Read the model definition and answer for the solid it produces. Units are mm, in the model's axes. A direction names the side the tool comes from. Coordinates: 2 decimals unless noted, no trailing zeros. Order: outer loops, then holes, each group sorted by start corner. A loop starts at its lowest first (then second) coordinate and runs counter-clockwise, first axis right, second up. Notation, with made-up numbers: M 35,-31 L 46,-31 A22 cw 46,-12 Z; hole C 45.5,68.5 d5. An arc over 180 degrees is marked long. Write each question's results on one line, items separated by ' | '.
```python
from build123d import *

# Parameters (mm, degrees)
BOSS_EXTRUDE1_DEPTH = 70
CUT_EXTRUDE1_DEPTH  = 65
SKETCH5_W           = 80
SKETCH5_H           = 35
BOSS_EXTRUDE2_DEPTH = 18
SKETCH6_W           = 70
SKETCH6_H           = 25
CUT_EXTRUDE2_DEPTH  = 18


with BuildPart() as part:
    # Sketch1 → Boss-Extrude1 (new body)
    with BuildSketch(Plane(origin=(0, 0, 0), x_dir=(1, 0, 0), z_dir=(0, 1, 0))):
        Polygon((-55.37403033, -102.482648945), (3.252686078, -116.449526131), (57.060212297, -100.408827863), (76.3, -57.735026919), (-76.3, -57.735026919), align=None)
    extrude(amount=BOSS_EXTRUDE1_DEPTH)

    # Sketch4 → Cut-Extrude1 (cut)
    with BuildSketch(Plane(origin=(0, 70, 0), x_dir=(1, 0, 0), z_dir=(0, 1, 0))):
        Polygon((-51.867290581, -98.178143042), (3.108154981, -111.275163368), (53.44146669, -96.270172009), (71.3, -57.735026919), (-71.3, -57.735026919), align=None)
    extrude(amount=-CUT_EXTRUDE1_DEPTH, mode=Mode.SUBTRACT)

    # Sketch5 → Boss-Extrude2 (add)
    with BuildSketch(Plane.XY.offset(117)):
        with Locations((3.252686078, 35)):
            Rectangle(SKETCH5_W, SKETCH5_H)
    extrude(amount=-BOSS_EXTRUDE2_DEPTH)

    # Sketch6 → Cut-Extrude2 (cut)
    with BuildSketch(Plane.XY.offset(117)):
        with Locations((3.252686078, 35)):
            Rectangle(SKETCH6_W, SKETCH6_H)
    extrude(amount=-CUT_EXTRUDE2_DEPTH, mode=Mode.SUBTRACT)


solid = part.part
```
(1) The part is cut by section A-A, the plane y = 28. Write down the section's boundary in (x, z).
Conclusion:
outline: M -76.3,57.74 L -71.3,57.74 L -51.87,98.18 L -36.75,101.78 L -36.75,99 L -31.75,99 L -31.75,117 L -36.75,117 L -36.75,106.92 L -55.37,102.48 Z; M 38.25,99 L 43.25,99 L 43.25,99.31 L 53.44,96.27 L 71.3,57.74 L 76.3,57.74 L 57.06,100.41 L 43.25,104.53 L 43.25,117 L 38.25,117 Z
(2) The mould has two halves that part along X. Classify faces 5 (the flat face through (47.7, 34.5, 103.2)), 6 (the flat face through (-39.499, 34.51, 106.265)), 7 (the flat face through (0, 22, 99)), 8 (the flat face through (62.246, 37.955, 77.272)): pulls with the +X half, pulls with the -X half, needs draft (parallel to the pull), parting line crosses it, or undercut.
Conclusion:
face 5: pulls with the +X half | face 6: pulls with the -X half | face 7: undercut | face 8: undercut
(3) For faces 1 (the flat face through (3, 52.5, 104)), 2 (the flat face through (3, 17.5, 104)), 3 (the flat face through (43.253, 35, 111)), 4 (the flat face through (3, 47.5, 108)), determine the directions among +Z, -Z, +X, -X, +Y, -Y from which every point of the face is accessible in a straight line to the end or side of a thin tool.
Conclusion:
face 1: -Z, +Y | face 2: -Z | face 3: +Z, +X, +Y, -Y | face 4: +Z, -Z
(4) The part is cut by section B-B, the plane x = 17.5. Write down the section's boundary in (y, z), then the cut area to 3 significant figures.
Conclusion:
outline: M 0,57.74 L 5,57.74 L 5,106.98 L 17.5,106.98 L 17.5,99 L 22.5,99 L 22.5,117 L 17.5,117 L 17.5,112.2 L 0,112.2 Z; M 47.5,99 L 52.5,99 L 52.5,106.98 L 70,106.98 L 70,112.2 L 52.5,112.2 L 52.5,117 L 47.5,117 Z | area: 609 mm²
(5) The part is cut by section C-C, the plane z = 109. Write down the section's boundary in (x, y).
Conclusion:
outline: M -36.75,17.5 L -28.02,17.5 L -28.02,0 L 28.24,0 L 28.24,17.5 L 43.25,17.5 L 43.25,52.5 L 28.24,52.5 L 28.24,70 L 10.74,70 L 10.74,52.5 L -6.44,52.5 L -6.44,70 L -28.02,70 L -28.02,52.5 L -36.75,52.5 Z; hole M -31.75,22.5 L 38.25,22.5 L 38.25,47.5 L -31.75,47.5 Z; hole M -6.44,5 L 10.74,5 L 10.74,17.5 L -6.44,17.5 Z
(6) The part is cut by section D-D, the plane y = 12. Write down the section's boundary in (x, z).
Conclusion:
outline: M -76.3,57.74 L -71.3,57.74 L -51.87,98.18 L 3.11,111.28 L 53.44,96.27 L 71.3,57.74 L 76.3,57.74 L 57.06,100.41 L 3.25,116.45 L -55.37,102.48 Z
(7) Straight lines are drawn through the part: line 1 (Y direction, x = 0, z = 105); line 2 (Y direction, x = 12, z = 112); line 3 (X direction, y = 40.5, z = 108). For each, find the intervals that lie inside material, in ascending order.
Conclusion:
line 1: 0 to 5, 17.5 to 22.5, 47.5 to 52.5 | line 2: 0 to 22.5, 47.5 to 70 | line 3: -36.75 to -31.75, 38.25 to 43.25
(8) Given pin 1 (6 mm diameter, centred on y = 32, z = 112, fed in from +X); pin 2 (1.5 mm diameter, centred on x = -15.5, z = 77.5, fed in from +Y); pin 3 (16 mm diameter, centred on x = -12, z = 95, fed in from +Y), each flat-ended and moving along its own axis, determine where each tip first touches the part or whether it passes through.
Conclusion:
pin 1: x = 43.25 | pin 2: y = 5 | pin 3: y = 52.5
